Part print with two shaded views. Sizes in mm from the minimum x, y, z corner. Give positions to 0.01 mm unless a question says otherwise; leave off trailing zeros. Order: outer loops, then holes, each group sorted by start corner. A loop starts at its lowest first (then second) coordinate and runs counter-clockwise, first axis right, second up.
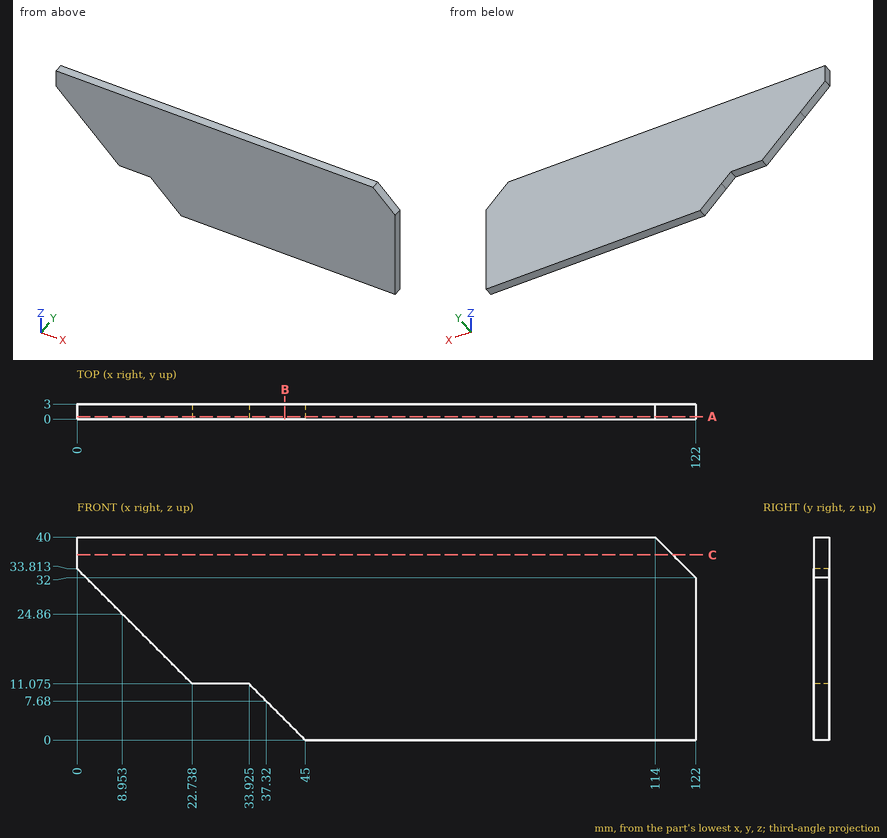
1. Saw through at A-A on y = 0.5. Give the cut face in (x, z) (1 decimal).
2. Saw through at C-C on z = 36.5. Give the cut face in (x, y).
3. Saw through at B-B on x = 41. Give the cut face in (y, z), plus the area to 3 significant figures.
4. Wall check: line 1 (Z direction, x = 31, y = 2.2) (1 decimal); line 2 (Z direction, x = 43, y = 1.85); line 3 (X direction, y = 2.05, z = 27) (1 decimal). Give the ranges that are in metal, low to high.
Reported:
1. outline: (0, 33.8) - (22.7, 11.1) - (33.9, 11.1) - (45, 0) - (122, 0) - (122, 32) - (114, 40) - (0, 40) - close
2. outline: (0, 0) - (117.5, 0) - (117.5, 3) - (0, 3) - close
3. outline: (0, 4) - (3, 4) - (3, 40) - (0, 40) - close
3. area: 108 mm2
4. line 1: z = 11.1 to 40
4. line 2: z = 2 to 40
4. line 3: x = 6.8 to 122
